Source: CAD feature listing. Evaluate the final solid. Frame: model axes, mm. Round coordinates to 2 decimals unless told otherwise and drop trailing zeros. Loops run counter-clockwise (first coordinate to the right, second up) from the corner with the lowest first, then second, coordinate; pieces in that order, holes last. Notation, with made-up numbers: (70, 38.5) -> (92, 38.5) arc R19 cw to (92, 72.5) -> close; hole circle Ø6 at (-25, -35.5). An arc over 180 degrees is marked (long way). Put each result on its own line as item: value. Start each with the question number.
1. Material intervals for L1, parallel to X at y = 4.7, z = -4.85, sorted ascending.
2. Contact query for flat-ended pins moving along their axis: pin 1 (1 mm diameter, centred on x = -1, z = -3.5, fed in from +Y); pin 2 (0.6 mm diameter, centred on x = -3, z = -3, fed in from -Y); pin 3 (0.6 mm diameter, centred on x = 204, y = 3.5, fed in from -Z). Output: stop coordinate, or through.
3. Cut plane A-A (z = -5). Return the cut outline in (x, y), then the cut area to 3 significant figures.
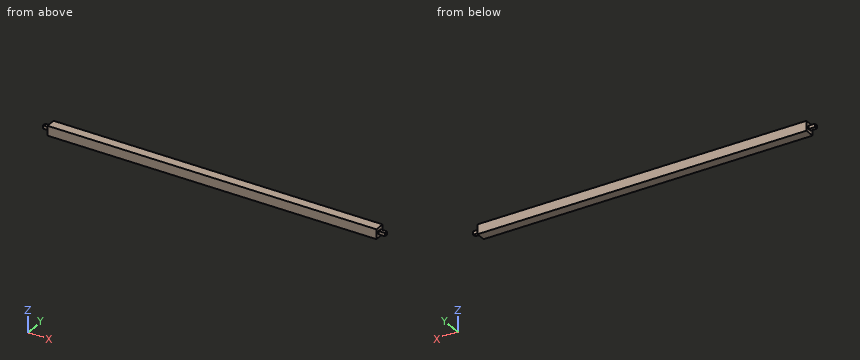
```python
from build123d import *

# Parameters (mm, degrees)
SKICA1_W                = 202
SKICA1_H                = 6
P_IDAT_VYSUNUT_M1_DEPTH = 6
SKICA2_W                = 2
SKICA2_H                = 2
P_IDAT_VYSUNUT_M2_DEPTH = 4
SKICA3_W                = 2
SKICA3_H                = 2
P_IDAT_VYSUNUT_M3_DEPTH = 4


with BuildPart() as part:
    # Skica1 → Přidat vysunutím1 (new body)
    with BuildSketch(Plane(origin=(0, 0, 0), x_dir=(1, 0, 0), z_dir=(0, 1, 0))):
        with Locations((101, 3)):
            Rectangle(SKICA1_W, SKICA1_H)
    extrude(amount=P_IDAT_VYSUNUT_M1_DEPTH)

    # Skica2 → Přidat vysunutím2 (add)
    with BuildSketch(Plane.ZY):
        with Locations((-3, 3)):
            Rectangle(SKICA2_W, SKICA2_H)
    extrude(amount=P_IDAT_VYSUNUT_M2_DEPTH)

    # Skica3 → Přidat vysunutím3 (add)
    with BuildSketch(Plane(origin=(202, 0, 0), x_dir=(0, 0, -1), z_dir=(1, 0, 0))):
        with Locations((3, 3)):
            Rectangle(SKICA3_W, SKICA3_H)
    extrude(amount=P_IDAT_VYSUNUT_M3_DEPTH)


solid = part.part
```
Solution:
1. L1: x = 0 to 202
2. pin 1: stops at y = 4
2. pin 2: stops at y = 2
2. pin 3: stops at z = -4
3. outline: (0, 0) -> (202, 0) -> (202, 6) -> (0, 6) -> close
3. area: 1,210 mm^2
